from build123d import *


with BuildPart() as part:
    # Sketch1 → Revolve1 (revolve)
    with BuildSketch(Plane.XY, mode=Mode.PRIVATE) as revolve1_sk:
        with BuildLine():
            Line((-15.367932956, -22.25), (11.632067044, -22.25))
            Line((11.632067044, -22.25), (11.632067044, -30))
            Line((11.632067044, -30), (11.132067044, -30))
            Line((11.132067044, -30), (11.132067044, -39.794883762))
            Line((11.132067044, -39.794883762), (-9.863295576, -39.794883762))
            Line((-9.863295576, -39.794883762), (-9.863295576, -35))
            Line((-9.863295576, -35), (-12.863295576, -35))
            Line((-12.863295576, -35), (-12.863295576, -39.936502505))
            Line((-12.863295576, -39.936502505), (-14.531334037, -39.936502505))
            Line((-14.531334037, -39.936502505), (-19.616831546, -39.794883762))
            Line((-19.616831546, -39.794883762), (-19.616831546, -38))
            Line((-19.616831546, -38), (-25.616831546, -38))
            Line((-25.616831546, -38), (-25.616831546, -40))
            Line((-25.616831546, -40), (-37.367932956, -39.794883762))
            Line((-37.367932956, -39.794883762), (-37.367932956, -33.332032388))
            Line((-37.367932956, -33.332032388), (-34.467915466, -33.332032388))
            Line((-34.467915466, -33.332032388), (-34.467915466, -34.832032388))
            Line((-34.467915466, -34.832032388), (-32.967915466, -34.832032388))
            Line((-32.967915466, -34.832032388), (-32.967915466, -33.332032388))
            Line((-32.967915466, -33.332032388), (-24.363295576, -33.332032388))
            ThreePointArc((-24.363295576, -33.332032388), (-22.241975232, -32.453352732), (-21.363295576, -30.332032388))
            Line((-21.363295576, -30.332032388), (-21.363295576, -23.24536262))
            Line((-21.363295576, -23.24536262), (-16.363295576, -23.24536262))
            ThreePointArc((-16.363295576, -23.24536262), (-15.659467917, -22.953827658), (-15.367932956, -22.25))
        make_face()
    revolve(revolve1_sk.sketch.rotate(Axis((-66.026476718, 0, 0), (1, 0, 0)), 270), axis=Axis((-66.026476718, 0, 0), (1, 0, 0)))


solid = part.part
Source: CAD feature listing. Evaluate the final solid. Frame: model axes, mm. A direction names the side the tool comes from. Coordinates: 2 decimals unless noted, no trailing zeros. Order: outer loops, then holes, each group sorted by start corner. A loop starts at its lowest first (then second) coordinate and runs counter-clockwise, first axis right, second up. Notation, with made-up numbers: M 37,73.5 L 60,73.5 A24 ccw 60,102.5 Z; hole C -14,-5.75 d9. An arc over 180 degrees is marked long. Write each question's results on one line, items separated by ' | '. Start each with the question number.
Item 1: Cut plane A-A (x = 6). Return loops of the section in (y, z).
Item 2: Set-up query: faces 1 (the face through (0.487, 38.849, -8.627)), 2 (the face through (-34.468, 2.4, -33.4)), 3 (the face through (-21.363, 18, 16)). Return all of +Z, -Z, +X, -X, +Y, -Y with unobstructed straight access to the full face (end or side cutting, diameter ignored); none if empty.
Item 3: Line query: probe 1 along X at (y, z) = (28, -22); probe 2 along Y at (x, z) = (-19.55, 0); probe 3 along Y at (x, z) = (-3.75, 0). Output: solid intervals per line, ascending.
Item 4: Draft query along Y for faces 4 (the face through (-18.24, -11.965, 37.994)), 5 (the face through (-12.863, 35.3, 0.2)), 6 (the face through (-28.61, 32.54, -7.23)), 7 (the face through (-18.828, -6.982, 22.172)). Return one class per face: pulls with the +Y half, pulls with the -Y half, needs draft (parallel to the pull), parting line crosses it, or undercut.
Item 5: First-contact query: pin 1 Ø3 at (y, z) = (-8.5, -30) entering from -X; pin 2 Ø8 at (y, z) = (-18.5, 14.5) entering from -X; pin 3 Ø1 at (x, z) = (-7, -12.5) entering from -Y. Flat tips, straight axial feed; report the tip coordinate or a pass-through.
Checked values:
1) outline: C 0,0 d79.59; hole C 0,0 d44.5
2) face 1: +X | face 2: none | face 3: -X
3) probe 1: x = -37.37 to -12.86, -9.86 to 11.13 | probe 2: y = -39.8 to -23.25, 23.25 to 39.8 | probe 3: y = -39.79 to -22.25, 22.25 to 39.79
4) face 4: parting line crosses it | face 5: needs draft | face 6: undercut | face 7: undercut
5) pin 1: stops at x = -22.5 | pin 2: stops at x = -21.36 | pin 3: stops at y = -37.94
